Print and shaded views of the part. All mm, measured from the part's lowest x, y and z. A direction names the side the tool comes from. Round coordinates to 2 decimals unless told otherwise and drop trailing zeros. Loops run counter-clockwise (first coordinate to the right, second up) from the corner with the lowest first, then second, coordinate; pieces in that order, holes last. Notation, with made-up numbers: (22, 71.5) - (41, 71.5) arc R24 cw to (41, 90.5) - close; hole circle Ø8 at (47, 33). An arc over 180 degrees is marked (long way). Use one line per item in the form item = value. Start each with the question number.
Q1. Saw through at A-A (z = 7.5). Give the cut face in (x, y) (3 decimals), then the cut area to 4 significant figures.
Q2. 3-axis set-ups, long thin cutter, end or side, ignore diameter. For the marked faces 1, 2 and 3: which of +Z, -Z, +X, -X, +Y, -Y reach the whole face in a straight line?
Q3. Saw through at C-C (y = 13.25). Give the cut face in (x, z) (3 decimals).
Q4. Pin check, flat tips, straight feed: pin 1 (4 mm diameter, centred on y = 12.5, z = 13, fed in from +X); pin 2 (2 mm diameter, centred on x = 9.5, y = 7, fed in from -Z); pin 3 (2 mm diameter, centred on x = 8, y = 15, fed in from +Z); pin 4 (7.5 mm diameter, centred on x = 7.5, z = 8, fed in from +Y). Stop position of each tip, or through.
Q5. Saw through at B-B (x = 7.5). Give the cut face in (y, z) (3 decimals).
Q6. Drill centre lines: line 1 (X direction, y = 11.25, z = 7.5) (3 decimals); line 2 (Y direction, x = 2.75, z = 2.5); line 3 (Z direction, x = 4, y = 1). Where is each one in solid material? Low to high.
Q7. Mould opens along X. For the marked faces 4, 5 and 6 say: released by +X, released by -X, zero draft, split by the parting line, or undercut.
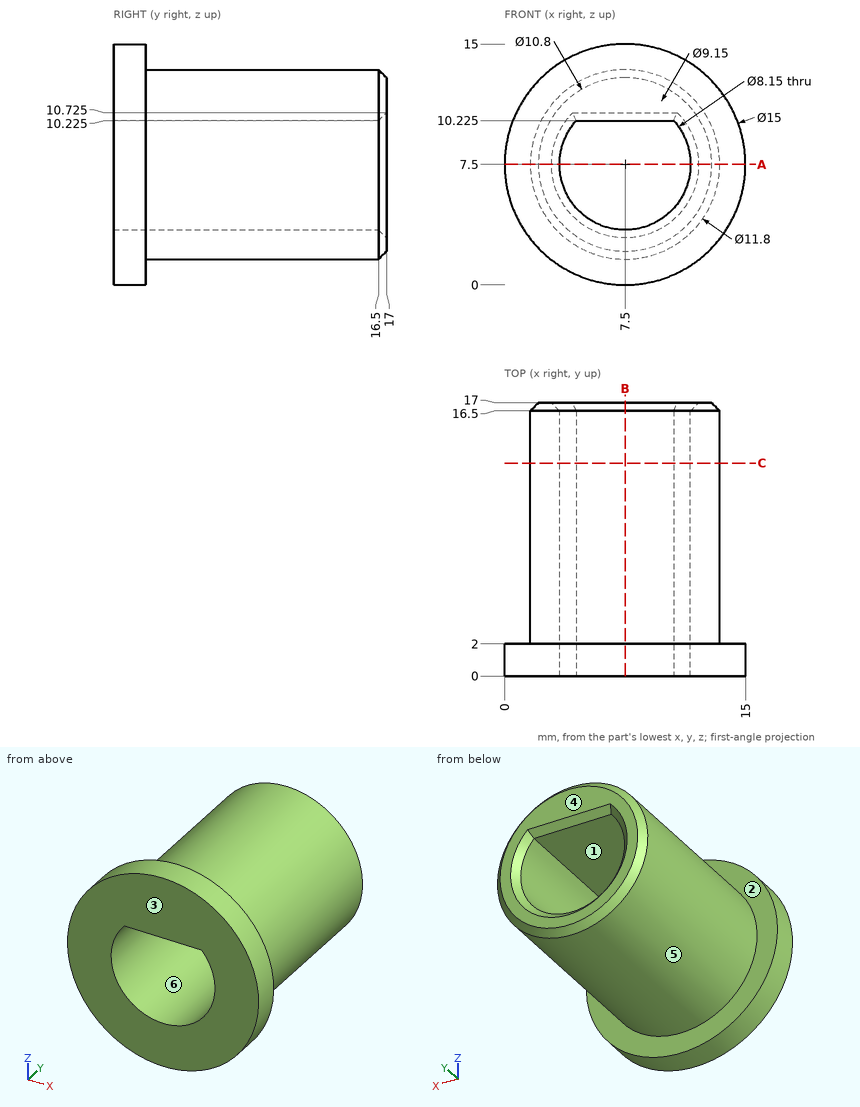
Report:
q1.outline = (0, 0) - (3.425, 0) - (3.425, 16.5) - (2.925, 17) - (2.1, 17) - (1.6, 16.5) - (1.6, 2) - (0, 2) - close; (11.575, 0) - (15, 0) - (15, 2) - (13.4, 2) - (13.4, 16.5) - (12.9, 17) - (12.075, 17) - (11.575, 16.5) - close
q1.area = 67.95 mm²
q2.face_1 = +Y, -Y
q2.face_2 = +Y
q2.face_3 = +Z, -Z, +X, -X, -Y
q3.outline = circle Ø11.8 at (7.5, 7.5); hole (4.47, 10.225) arc R4.075 ccw (long way) to (10.53, 10.225) - close
q4.pin_1 = 12.25
q4.pin_2 = 1.69
q4.pin_3 = 13.4
q4.pin_4 = 17
q5.outline = (0, 0) - (2, 0) - (2, 1.6) - (16.5, 1.6) - (17, 2.1) - (17, 2.925) - (16.5, 3.425) - (0, 3.425) - close; (0, 10.225) - (16.5, 10.225) - (17, 10.725) - (17, 12.9) - (16.5, 13.4) - (2, 13.4) - (2, 15) - (0, 15) - close
q6.line_1 = 1.6 to 3.425, 11.575 to 13.4
q6.line_2 = 0 to 2
q6.line_3 = 0.87 to 5.41, 9.59 to 14.13
q7.face_4 = zero draft
q7.face_5 = split by the parting line
q7.face_6 = undercut
